Here's the drawing with two shaded views (mm, measured from the low corner). I have some questions. A direction names the side the tool comes from. Coordinates: 2 decimals unless noted, no trailing zeros. Loops run counter-clockwise (first coordinate to the right, second up) from the corner with the lowest first, then second, coordinate; pieces in that order, holes last. Notation, with made-up numbers: (46.5, 89.5) -> (86.5, 89.5) arc R17 cw to (86.5, 115.5) -> close; hole circle Ø4 at (89, 34.25). An arc over 180 degrees is marked (long way). Answer as a JSON object with one key per item and string values. Group by question number.
1) I'm going to push flat-ended pins straight in: pin 1 (2 mm diameter, centred on x = 4, y = 5, fed in from -Z); pin 2 (2.5 mm diameter, centred on x = 10, y = 10, fed in from -Z); pin 3 (2 mm diameter, centred on x = 6, z = 4.5, fed in from +Y); pin 4 (2 mm diameter, centred on x = 5, z = 8, fed in from +Y). Where does each tip first touch, or does it pass through?
2) I want a section at A-A (y = 10). Write out the boundary of the cut face in (x, z), then the cut area to 3 significant figures.
3) Which directions (+Z, -Z, +X, -X, +Y, -Y) give clear straight access to the entire face, cutting with the end or side of a thin tool? Please do the marked faces 1 and 2.
4) If we mould it in two halves opening along Y, with no side actions, what happens to the marked faces 3, 4 and 5? For each: +Y half, -Y half, draft (parallel to the pull), parting line (faces both ways), or undercut.
5) I want a section at D-D (z = 3). Write out the boundary of the cut face in (x, y), then the cut area to 3 significant figures.
6) I want a section at B-B (z = 6.25). Write out the boundary of the cut face in (x, y), then the cut area to 3 significant figures.
7) I need wall thicknesses on probe 1 along Y at (x, z) = (10, 4); probe 2 along Z at (x, y) = (3.5, 14.5); probe 3 along Y at (x, z) = (9.5, 3.5) (3 decimals). Which ranges of each line are inside material? Lowest first, please. Write a range as [from, to].
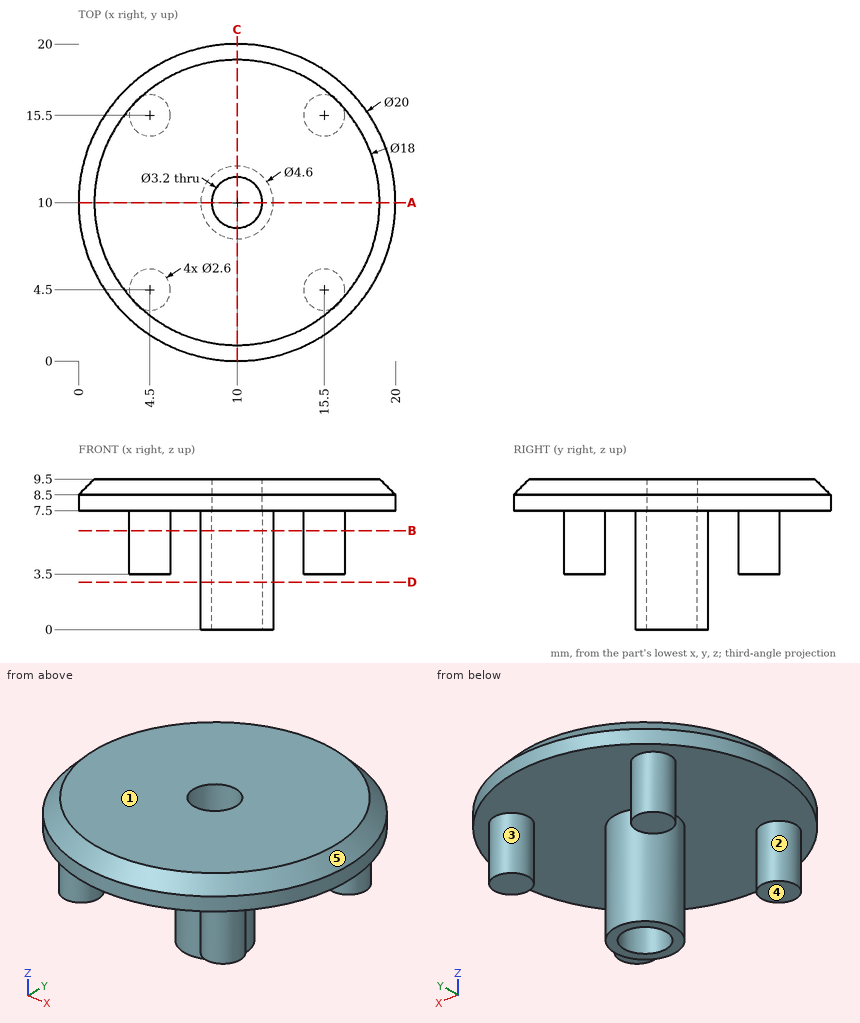
Determined:
{
 "1": {"pin 1": "z = 3.5", "pin 2": "through", "pin 3": "y = 16.7", "pin 4": "y = 19.17"},
 "2": {"outline": "(0, 7.5) -> (7.7, 7.5) -> (7.7, 0) -> (8.4, 0) -> (8.4, 9.5) -> (1, 9.5) -> (0, 8.5) -> close; (11.6, 0) -> (12.3, 0) -> (12.3, 7.5) -> (20, 7.5) -> (20, 8.5) -> (19, 9.5) -> (11.6, 9.5) -> close", "area": "43.1 mm^2"},
 "3": {"face 1": "+Z, +X, -X, +Y, -Y", "face 2": "-Z"},
 "4": {"face 3": "undercut", "face 4": "draft", "face 5": "parting line"},
 "5": {"outline": "circle Ø4.6 at (10, 10); hole circle Ø3.2 at (10, 10)", "area": "8.58 mm^2"},
 "6": {"outline": "circle Ø2.6 at (4.5, 4.5); circle Ø2.6 at (4.5, 15.5); circle Ø4.6 at (10, 10); circle Ø2.6 at (15.5, 4.5); circle Ø2.6 at (15.5, 15.5); hole circle Ø3.2 at (10, 10)", "area": "29.8 mm^2"},
 "7": {"probe 1": "[7.7, 8.4], [11.6, 12.3]", "probe 2": "[7.5, 9.5]", "probe 3": "[7.755, 8.48], [11.52, 12.245]"}
}
